Answer from the drawing. Dimensions are ordinates in mm from the lowest x, y and z of the part. Round coordinates to 2 decimals unless told otherwise and drop trailing zeros. Order: outer loops, then holes, each group sorted by start corner. A loop starts at its lowest first (then second) coordinate and runs counter-clockwise, first axis right, second up. Notation, with made-up numbers: (89, 52.5) -> (95, 52.5) arc R28 ccw to (95, 82.5) -> close; hole circle Ø5 at (65.5, 88). An arc over 180 degrees is marked (long way). Use a Markdown table: item, result. Add a question column.
Item 1: A cutting plane is placed at C-C, the plane y = 5.5. Determine the outline of the cut face in (x, z), plus the area to 3 significant figures.
Item 2: A cutting plane is placed at B-B, the plane x = 30. Determine the outline of the cut face in (y, z).
Item 3: A cutting plane is placed at A-A, the plane z = 30. Determine the outline of the cut face in (x, y).
Item 4: For a pull along X with two mould halves and no side action, classify the marked faces 1, 2 and 3 as +X half, -X half, draft (parallel to the pull), parting line (faces both ways), or undercut.
Item 5: Flat-ended cylindrical pins translate along their axes: P1, Ø1, axis at x = 24, z = 11.5, coming from the -Y side; P2, Ø18, axis at x = 30, z = 30, coming from the -Y side. Find the tip coordinate at first contact, or state that the pin passes through.
Item 6: Find the intervals of material crossed by L1, parallel to Z at x = 30, y = 35; L2, parallel to X at y = 12.5, z = 29.5; L3, parallel to X at y = 38, z = 27, in increasing order. Write a range as [from, to].
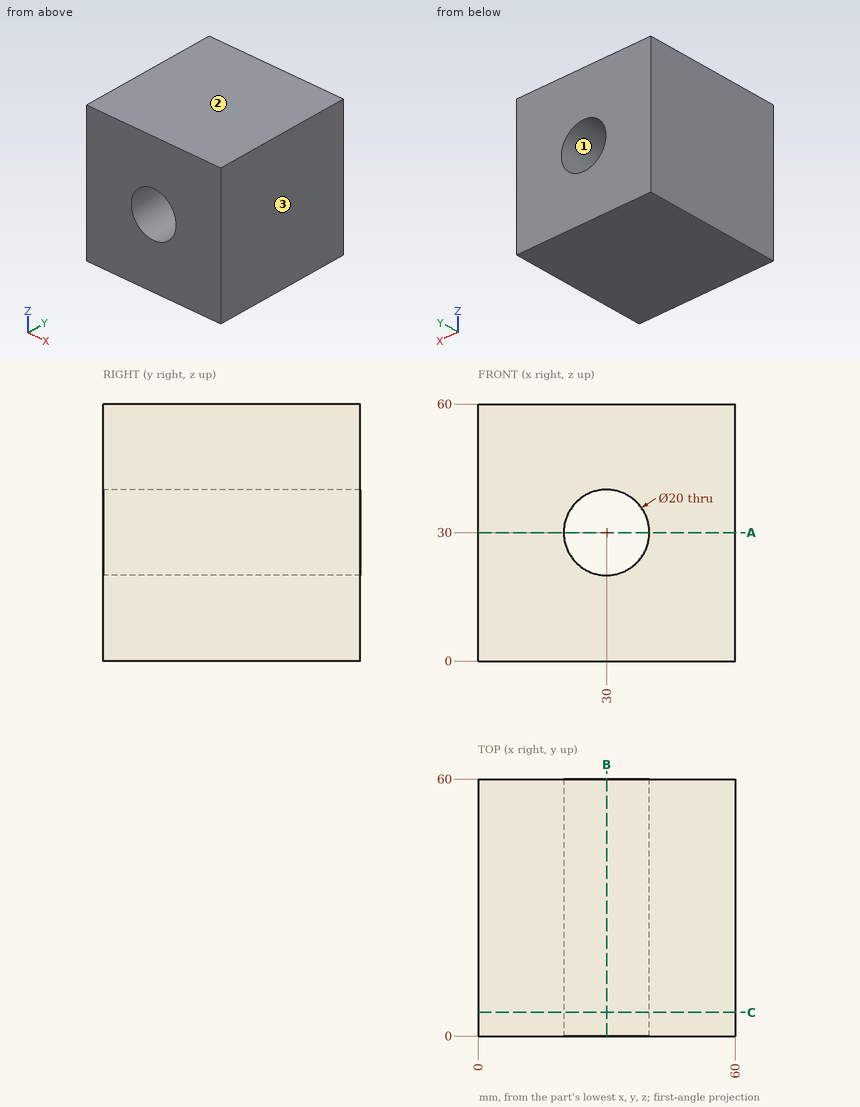
Reported:
| question | item | result |
|---|---|---|
| 1 | outline | (0, 0) -> (60, 0) -> (60, 60) -> (0, 60) -> close; hole circle Ø20 at (30, 30) |
| 1 | area | 3,290 mm² |
| 2 | outline | (0, 0) -> (60, 0) -> (60, 20) -> (0, 20) -> close; (0, 40) -> (60, 40) -> (60, 60) -> (0, 60) -> close |
| 3 | outline | (0, 0) -> (20, 0) -> (20, 60) -> (0, 60) -> close; (40, 0) -> (60, 0) -> (60, 60) -> (40, 60) -> close |
| 4 | face 1 | undercut |
| 4 | face 2 | draft |
| 4 | face 3 | +X half |
| 5 | P1 | y = 0 |
| 5 | P2 | through |
| 6 | L1 | [0, 20], [40, 60] |
| 6 | L2 | [0, 20.01], [39.99, 60] |
| 6 | L3 | [0, 20.46], [39.54, 60] |
